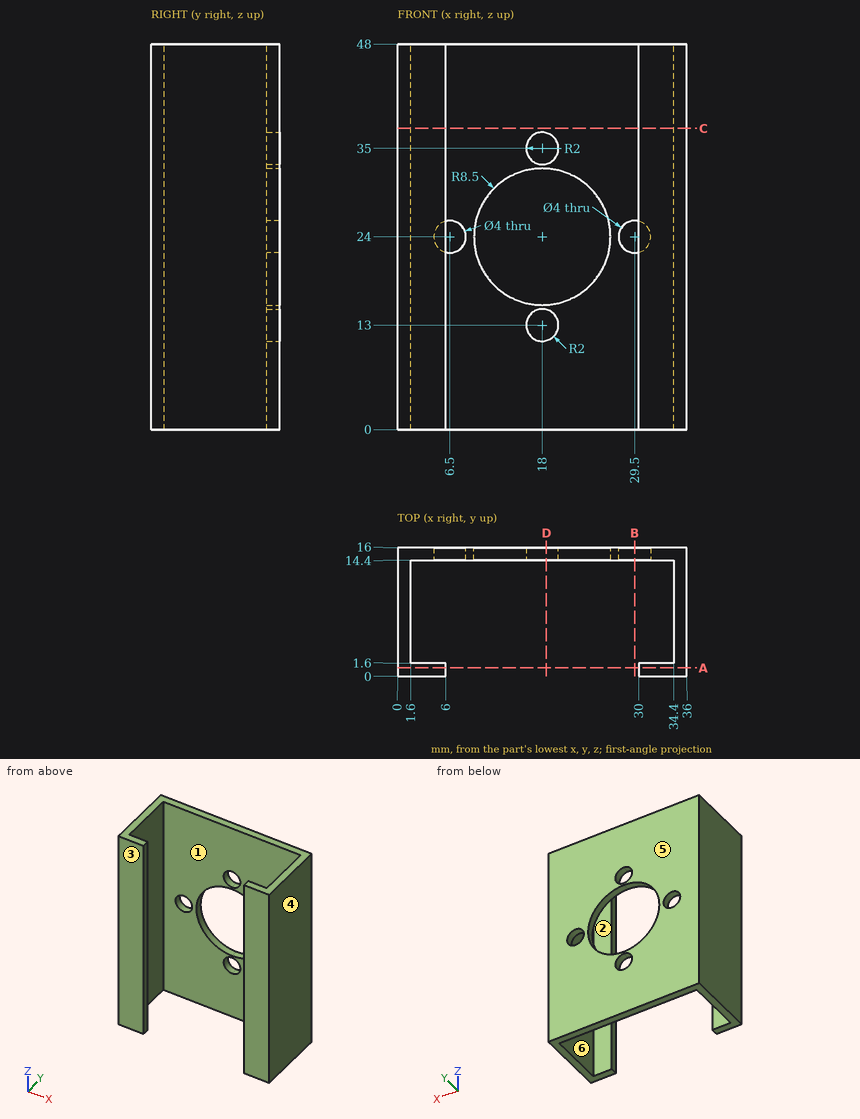
Can you work these out from the drawing? Everything is in mm from the part's minimum corner. A direction names the side the tool comes from. Give positions to 0.01 mm unless a question says otherwise; leave off trailing zeros. Order: outer loops, then holes, each group sorted by start corner. A loop starts at its lowest first (then second) coordinate and runs counter-clockwise, first axis right, second up.
Item 1: If we section it at B-B, the plane x = 29.5: Write out the boundary of the cut face in (y, z).
Item 2: If we section it at D-D, the plane x = 18.5: Write out the boundary of the cut face in (y, z).
Item 3: If we section it at A-A, the plane y = 1: Write out the boundary of the cut face in (x, z), plus the area to 3 significant figures.
Item 4: I need wall thicknesses on line 1 (X direction, y = 8.5, z = 29); line 2 (Z direction, x = 6.5, y = 15); line 3 (Y direction, x = 32.5, z = 21). Which ranges of each line are inside material? Lowest first, please.
Item 5: I'm going to push flat-ended pins straight in: pin 1 (2.5 mm diameter, centred on x = 29.5, z = 24, fed in from +Y); pin 2 (4 mm diameter, centred on x = 10, z = 20, fed in from -Y); pin 3 (3 mm diameter, centred on x = 15, y = 11.5, fed in from +Z). Where does each tip first touch, or does it pass through?
Item 6: If we section it at C-C, the plane z = 37.5: Write out the boundary of the cut face in (x, y), plus the area to 3 significant figures.
Item 7: If we mould it in two halves opening along X, with no side actions, what happens to the marked faces 1, 2, 3 and 4? For each: pulls with the +X half, pulls with the -X half, needs draft (parallel to the pull), parting line crosses it, or undercut.
Item 8: For the marked faces 5 and 6, which set-ups out of +Z, -Z, +X, -X, +Y, -Y let a thin tool reach every point of the face, with its end or its side?
Values:
1. outline: (14.4, 0) - (16, 0) - (16, 22) - (14.4, 22) - close; (14.4, 26) - (16, 26) - (16, 48) - (14.4, 48) - close
2. outline: (14.4, 0) - (16, 0) - (16, 11.06) - (14.4, 11.06) - close; (14.4, 14.94) - (16, 14.94) - (16, 15.51) - (14.4, 15.51) - close; (14.4, 32.49) - (16, 32.49) - (16, 33.06) - (14.4, 33.06) - close; (14.4, 36.94) - (16, 36.94) - (16, 48) - (14.4, 48) - close
3. outline: (0, 0) - (6, 0) - (6, 48) - (0, 48) - close; (30, 0) - (36, 0) - (36, 48) - (30, 48) - close
3. area: 576 mm2
4. line 1: x = 0 to 1.6, 34.4 to 36
4. line 2: z = 0 to 22, 26 to 48
4. line 3: y = 0 to 1.6, 14.4 to 16
5. pin 1: stops at y = 1.6
5. pin 2: stops at y = 14.4
5. pin 3: passes through
6. outline: (0, 0) - (6, 0) - (6, 1.6) - (1.6, 1.6) - (1.6, 14.4) - (34.4, 14.4) - (34.4, 1.6) - (30, 1.6) - (30, 0) - (36, 0) - (36, 16) - (0, 16) - close
6. area: 118 mm2
7. face 1: undercut
7. face 2: undercut
7. face 3: needs draft
7. face 4: pulls with the +X half
8. face 5: +Z, -Z, +X, -X, +Y
8. face 6: +Z, -Z
